Part model, mm, in its own coordinate system. A direction names the side the tool comes from. Coordinates: 2 decimals unless noted, no trailing zeros. Order: outer loops, then holes, each group sorted by start corner. A loop starts at its lowest first (then second) coordinate and runs counter-clockwise, first axis right, second up.
from build123d import *

# Parameters (mm, degrees)
SKETCH_1_R          = 10
EXTRUDE_1_DEPTH     = 2
SKETCH_2_R          = 2.5
EXTRUDE_2_DEPTH     = 35
SKETCH_3_R          = 1
SKETCH_3_R_2        = 0.75
CUT_EXTRUDE_1_DEPTH = 3
SKETCH_4_R          = 3.5
CUT_EXTRUDE_2_DEPTH = 1
SKETCH_6_R          = 4
EXTRUDE_4_DEPTH     = 3
CUT_EXTRUDE_START   = -26
CUT_EXTRUDE_3_DEPTH = 20
SKETCH_12_R         = 1.1
CUT_EXTRUDE_6_DEPTH = 3


with BuildPart() as part:
    # 草图1 → 凸台-拉伸1 (new body)
    with BuildSketch(Plane(origin=(0, 0, 0), x_dir=(1, 0, 0), z_dir=(0, 1, 0))):
        with Locations(Location((0, 0, 0), (0, 0, 270))):
            Circle(SKETCH_1_R)
    extrude(amount=EXTRUDE_1_DEPTH)

    # 草图2 → 凸台-拉伸2 (add)
    with BuildSketch(Plane(origin=(0, 2, 0), x_dir=(1, 0, 0), z_dir=(0, 1, 0))):
        with Locations(Location((0, 0, 0), (0, 0, 270))):
            Circle(SKETCH_2_R)
    extrude(amount=EXTRUDE_2_DEPTH)

    # 草图3 → 切除-拉伸1 (cut)
    with BuildSketch(Plane.XZ):
        with Locations(Location((-3.15926406, 5.68058541, 0), (0, 0, 270))):
            Circle(SKETCH_3_R)
        with Locations(Location((3.15926406, -5.68058541, 0), (0, 0, 90))):
            Circle(SKETCH_3_R)
        with Locations(Location((5.121266231, 2.84819806, 0), (0, 0, 270))):
            Circle(SKETCH_3_R_2)
        with Locations(Location((-5.121266231, -2.84819806, 0), (0, 0, 90))):
            Circle(SKETCH_3_R_2)
    extrude(amount=-CUT_EXTRUDE_1_DEPTH, mode=Mode.SUBTRACT)

    # 草图4 → 切除-拉伸2 (cut)
    with BuildSketch(Plane.XZ):
        with Locations(Location((0, 0, 0), (0, 0, 270))):
            Circle(SKETCH_4_R)
    extrude(amount=-CUT_EXTRUDE_2_DEPTH, mode=Mode.SUBTRACT)

    # 草图6 → 凸台-拉伸4 (add)
    with BuildSketch(Plane(origin=(0, 2, 0), x_dir=(1, 0, 0), z_dir=(0, 1, 0))):
        with Locations(Location((0, 0, 0), (0, 0, 270))):
            Circle(SKETCH_6_R)
    extrude(amount=EXTRUDE_4_DEPTH)

    # 草图7 → 切除-拉伸3 (cut)
    with BuildSketch(Plane(origin=(0, 37, 0), x_dir=(1, 0, 0), z_dir=(0, 1, 0)).offset(CUT_EXTRUDE_START)):
        with BuildLine():
            Line((2.157730635, 1.26261574), (-2.157730635, -1.26261574))
            ThreePointArc((-2.157730635, -1.26261574), (-1.26261574, 2.157730635), (2.157730635, 1.26261574))
        make_face()
    extrude(amount=CUT_EXTRUDE_3_DEPTH, mode=Mode.SUBTRACT)

    # 草图12 → 切除-拉伸6 (cut)
    with BuildSketch(Plane(origin=(0, 0, 0), x_dir=(-0.8630922540018389, 0, 0.5050462959789186), z_dir=(-0.5050462959789186, 0, -0.8630922540018389))):
        with Locations((0, 16.5)):
            Circle(SKETCH_12_R)
    cut_extrude_6 = extrude(amount=-CUT_EXTRUDE_6_DEPTH, mode=Mode.SUBTRACT)

    # 镜向1: 切除-拉伸6 across plane
    add(cut_extrude_6.mirror(Plane.ZX.offset(21)), mode=Mode.SUBTRACT)


solid = part.part
Q1. Mould opens along Z. For faces 6 (the face through (-5.347, 0.986, -2.133)), 7 (the face through (2.11, 20.78, 1.34)), 8 (the face through (0, 0, 4)) say: pulls with the +Z half, pulls with the -Z half, needs draft (parallel to the pull), parting line crosses it, or undercut.
Results list:
face 6: undercut
face 7: parting line crosses it
face 8: needs draft
Q2. Pin check, flat tips, straight feed: pin 1 Ø3.5 at (x, z) = (-1, 1) entering from -Y; pin 2 Ø12 at (x, y) = (-4.5, 26.5) entering from -Z; pin 3 Ø1.7 at (x, z) = (-5.12, -2.85) entering from +Y. Stop position of each tip, or through.
Results list:
pin 1: stops at y = 1
pin 2: stops at z = -2.44
pin 3: stops at y = 2
Q3. Cut at D-D on z = -9. Write the cut outline in (x, y), and give its area (3 significant figures).
Results list:
outline: (-4.36, 0) - (4.36, 0) - (4.36, 2) - (-4.36, 2) - close
area: 17.4 mm2
Q4. Cut at A-A on z = 6. Write the cut outline in (x, y), and give its area (3 significant figures).
Results list:
outline: (-8, 0) - (-4.11, 0) - (-4.11, 2) - (-8, 2) - close; (-2.21, 0) - (8, 0) - (8, 2) - (-2.21, 2) - close
area: 28.2 mm2
Q5. Cut at B-B on y = 10. Write the cut outline in (x, z).
Results list:
outline: circle Ø5 at (0, 0)
Q6. Which spindle directions (+Z, -Z, +X, -X, +Y, -Y) get a long thin tool onto all of the face, cutting with end or side? Do faces 1 (the face through (0, 37, 0)), 2 (the face through (-3.417, 0.493, 0.759)), 3 (the face through (0, 21, 0)), 4 (the face through (-3.905, 3.479, -0.867)), 5 (the face through (5.347, 0.986, 2.133)). Say none if no direction does.
Results list:
face 1: +Z, -Z, +X, -X, +Y
face 2: -Y
face 3: -Z, -X
face 4: +Y
face 5: +Y, -Y
Q7. Wall check: line 1 along Y through (x, z) = (2, -1.25); line 2 along Y through (x, z) = (-1.5, -4); line 3 along X through (y, z) = (0.8, 0). Give the ranges that are in metal, low to high.
Results list:
line 1: y = 1 to 11, 31 to 37
line 2: y = 0 to 2
line 3: x = -10 to -3.5, 3.5 to 10
Q8. Cut at C-C on x = -6.5. Write the cut outline in (y, z).
Results list:
outline: (0, -7.6) - (2, -7.6) - (2, 7.6) - (0, 7.6) - close
